Build history of the part. All positions in model axes, mm. Give positions to 0.01 mm unless a question says otherwise; leave off trailing zeros. Write each loop counter-clockwise with the first axis right and the second up, starting at its lowest first coordinate (ties: lowest second). Pieces come first, ordered by that corner, then holes. Notation, with made-up numbers: (25.5, 1.25) -> (49.5, 1.25) arc R17 ccw to (49.5, 13.25) -> close; hole circle Ø4 at (-8, -8.75). An arc over 180 degrees is marked (long way). Put each result on its own line as item: value. Start each with the question number.
Item 1: Slice it at A-A, the plane y = 3.35. Give the number of separate pieces and of enclosed holes in the cut face, plus the area to 3 significant figures.
Item 2: Drill centre lines: line 1 along X through (y, z) = (2.9, 29.5); line 2 along Z through (x, y) = (-17.5, 1.9); line 3 along Z through (x, y) = (159, 1.2). Where is each one in solid material? Low to high.
Item 3: Flat gauge pins, fed straight in: pin 1 Ø2.5 at (y, z) = (2, 97) entering from +X; pin 2 Ø0.9 at (x, y) = (-167, 2.5) entering from +Z; pin 3 Ø1.5 at (x, y) = (13, 1) entering from +Z. Where does each tip first touch, or does it go through?
Item 4: Slice it at C-C, the plane x = 145. List the corners of the cut face in (y, z).
Item 5: Slice it at B-B, the plane z = -90.5. List the corners of the cut face in (x, y).
```python
from build123d import *

# Parameters (mm, degrees)
SKETCH1_W           = 3
SKETCH1_H           = 15.635202888
SKETCH1_H_2         = 15.6
SKETCH1_H_3         = 15.635202889
BOSS_EXTRUDE1_DEPTH = 5


with BuildPart() as part:
    # Sketch1 → Boss-Extrude1 (new body)
    with BuildSketch(Plane(origin=(0, 0, 0), x_dir=(1, 0, 0), z_dir=(0, 1, 0))):
        with BuildLine():
            Line((-30.000015974, -136.250310986), (-18.000015974, -136.250310986))
            Line((-18.000015974, -136.250310986), (-18.000015974, -131.250310986))
            Line((-18.000015974, -131.250310986), (-6.000015974, -131.250310986))
            Line((-6.000015974, -131.250310986), (-6.000015974, -136.250310986))
            Line((-6.000015974, -136.250310986), (5.999984026, -136.250310986))
            Line((5.999984026, -136.250310986), (5.999984026, -131.250310986))
            Line((5.999984026, -131.250310986), (17.999984026, -131.250310986))
            Line((17.999984026, -131.250310986), (17.999984026, -136.250310986))
            Line((17.999984026, -136.250310986), (30.000006721, -136.250310986))
            Line((30.000006721, -136.250310986), (30.000006721, -116.24999063))
            ThreePointArc((30.000006721, -116.24999063), (32.92893891, -109.178922818), (40.000006721, -106.24999063))
            Line((40.000006721, -106.24999063), (36.229984025, -106.24999063))
            Line((36.229984025, -106.24999063), (36.229984025, -103.249670275))
            Line((36.229984025, -103.249670275), (108.689984025, -103.249670275))
            Line((108.689984025, -103.249670275), (108.689984025, -106.24999063))
            Line((108.689984025, -106.24999063), (181.149984025, -106.24999063))
            Line((181.149984025, -106.24999063), (181.149984025, -103.24999063))
            Line((181.149984025, -103.24999063), (178.149984476, -103.24999063))
            Line((178.149984476, -103.24999063), (178.149984476, -61.94999063))
            Line((178.149984476, -61.94999063), (181.149984025, -61.94999063))
            Line((181.149984025, -61.94999063), (181.149984025, -20.64999063))
            Line((181.149984025, -20.64999063), (178.149984927, -20.64999063))
            Line((178.149984927, -20.64999063), (178.149984927, 20.65000937))
            Line((178.149984927, 20.65000937), (181.149984025, 20.65000937))
            Line((181.149984025, 20.65000937), (181.149984025, 61.95000937))
            Line((181.149984025, 61.95000937), (178.149984927, 61.95000937))
            Line((178.149984927, 61.95000937), (178.149984927, 103.25000937))
            Line((178.149984927, 103.25000937), (181.149984025, 103.25000937))
            Line((181.149984025, 103.25000937), (181.150047924, 106.25000937))
            Line((181.150047924, 106.25000937), (108.689984025, 106.25000937))
            Line((108.689984025, 106.25000937), (108.689984025, 103.249689014))
            Line((108.689984025, 103.249689014), (36.229984025, 103.249689014))
            Line((36.229984025, 103.249689014), (36.229984025, 106.25000937))
            Line((36.229984025, 106.25000937), (-36.230015974, 106.25000937))
            Line((-36.230015974, 106.25000937), (-36.230015974, 103.249689014))
            Line((-36.230015974, 103.249689014), (-108.690015974, 103.249689014))
            Line((-108.690015974, 103.249689014), (-108.690015974, 106.25000937))
            Line((-108.690015974, 106.25000937), (-181.150015974, 106.25000937))
            Line((-181.150015974, 106.25000937), (-181.150015974, 103.25000937))
            Line((-181.150015974, 103.25000937), (-178.150016876, 103.25000937))
            Line((-178.150016876, 103.25000937), (-178.150016876, 61.95000937))
            Line((-178.150016876, 61.95000937), (-181.150015974, 61.95000937))
            Line((-181.150015974, 61.95000937), (-181.150015974, 20.65000937))
            Line((-181.150015974, 20.65000937), (-178.150016876, 20.65000937))
            Line((-178.150016876, 20.65000937), (-178.150016876, -20.64999063))
            Line((-178.150016876, -20.64999063), (-181.150015974, -20.64999063))
            Line((-181.150015974, -20.64999063), (-181.150015974, -61.94999063))
            Line((-181.150015974, -61.94999063), (-178.150016425, -61.94999063))
            Line((-178.150016425, -61.94999063), (-178.150016425, -103.24999063))
            Line((-178.150016425, -103.24999063), (-181.150015974, -103.24999063))
            Line((-181.150015974, -103.24999063), (-181.150015974, -106.24999063))
            Line((-181.150015974, -106.24999063), (-108.690015974, -106.24999063))
            Line((-108.690015974, -106.24999063), (-108.690015974, -103.24999063))
            Line((-108.690015974, -103.24999063), (-111.150015974, -103.24999063))
            Line((-111.150015974, -103.24999063), (-111.150015974, -100.24999063))
            Line((-111.150015974, -100.24999063), (-81.150015974, -100.24999063))
            Line((-81.150015974, -100.24999063), (-81.150015974, -103.249670275))
            Line((-81.150015974, -103.249670275), (-36.230015974, -103.249670275))
            Line((-36.230015974, -103.249670275), (-36.230015974, -106.24999063))
            Line((-36.230015974, -106.24999063), (-40.000015974, -106.24999063))
            ThreePointArc((-40.000015974, -106.24999063), (-32.928948162, -109.178922818), (-30.000015974, -116.24999063))
            Line((-30.000015974, -116.24999063), (-30.000015974, -136.250310986))
        make_face()
        with Locations((-166.650000226, -95.537975278)):
            Rectangle(SKETCH1_W, SKETCH1_H, mode=Mode.SUBTRACT)
        with Locations((-16.650016425, -95.449968057)):
            Rectangle(SKETCH1_W, SKETCH1_H_2, mode=Mode.SUBTRACT)
        with Locations((-166.650000226, -32.997163725)):
            Rectangle(SKETCH1_W, SKETCH1_H, mode=Mode.SUBTRACT)
        with Locations((-16.650016425, -33.049968057)):
            Rectangle(SKETCH1_W, SKETCH1_H_2, mode=Mode.SUBTRACT)
        with Locations((-166.650000226, -64.267569502)):
            Rectangle(SKETCH1_W, SKETCH1_H_3, mode=Mode.SUBTRACT)
        with Locations((-16.650016425, -64.249968057)):
            Rectangle(SKETCH1_W, SKETCH1_H_2, mode=Mode.SUBTRACT)
    extrude(amount=BOSS_EXTRUDE1_DEPTH)


solid = part.part
```
Values follow:
1. separate pieces: 1
1. enclosed holes: 6
1. area: 76,700 mm2
2. line 1: -181.15 to -168.15, -165.15 to -18.15, -15.15 to 181.15
2. line 2: -106.25 to 25.25, 40.85 to 56.45, 72.05 to 87.65, 103.25 to 131.25
2. line 3: -106.25 to 106.25
3. pin 1: x = 178.15
3. pin 2: z = 106.25
3. pin 3: z = 131.25
4. outline: (0, -106.25) -> (5, -106.25) -> (5, 106.25) -> (0, 106.25) -> close
5. outline: (-178.15, 0) -> (178.15, 0) -> (178.15, 5) -> (-178.15, 5) -> close
